from build123d import *

# Parameters (mm, degrees)
SALIENTE_EXTRUIR1_DEPTH                              = 15
CROQUIS2_R                                           = 1.5
CORTAR_EXTRUIR1_DEPTH                                = 5
AVELLANADO_PARA_TORNILLO_CON_CABEZA_PLAN_D           = 3.4
AVELLANADO_PARA_TORNILLO_CON_CABEZA_PLAN_CSINK_D     = 6.3
AVELLANADO_PARA_TORNILLO_CON_CABEZA_PLAN_CSINK_ANGLE = 90


with BuildPart() as part:
    # Croquis1 → Saliente-Extruir1 (new body)
    with BuildSketch(Plane.XY):
        Polygon((-24.277819577, -18.779195804), (-24.277819577, -23.779195804), (-44.277819577, -23.779195804), (-44.277819577, 10.220804196), (-84.277819577, 10.220804196), (-84.277819577, 12.320804196), (-42.177819577, 12.320804196), (-42.177819577, -18.779195804), align=None)
    extrude(amount=SALIENTE_EXTRUIR1_DEPTH)

    # Croquis2 → Cortar-Extruir1 (cut)
    with BuildSketch(Plane(origin=(0, -18.779195804, 0), x_dir=(1, 0, 0), z_dir=(0, 1, 0))):
        with Locations((-33.227819577, -7.5)):
            Circle(CROQUIS2_R)
    extrude(amount=-CORTAR_EXTRUIR1_DEPTH, mode=Mode.SUBTRACT)

    # Avellanado para tornillo con cabeza plana avellanada de M31 (through all)
    with Locations(Plane(origin=(0, -18.779195804, 0), x_dir=(1, 0, 0), z_dir=(0, 1, 0))):
        with Locations((-33.227819577, -7.5)):
            CounterSinkHole(AVELLANADO_PARA_TORNILLO_CON_CABEZA_PLAN_D / 2, AVELLANADO_PARA_TORNILLO_CON_CABEZA_PLAN_CSINK_D / 2, counter_sink_angle=AVELLANADO_PARA_TORNILLO_CON_CABEZA_PLAN_CSINK_ANGLE)


solid = part.part
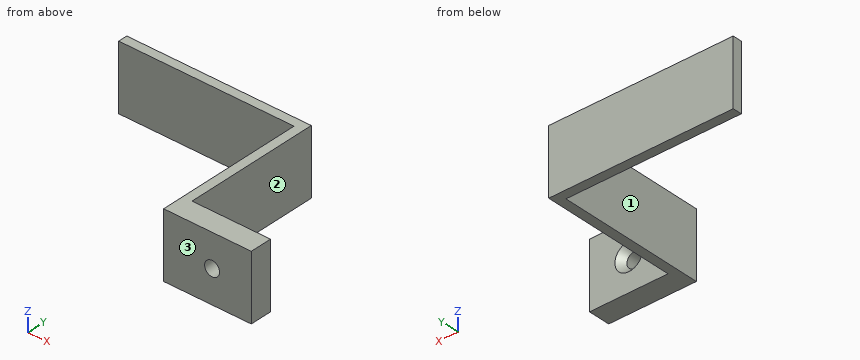
CAD build for the part. Positions are in the model's coordinates, mm. Face numbers are marked on the shaded views. A direction names the side the tool comes from. Give positions to 0.01 mm unless a question says otherwise; leave off trailing zeros. Order: outer loops, then holes, each group sorted by start corner. A loop starts at its lowest first (then second) coordinate and runs counter-clockwise, first axis right, second up. Notation, with made-up numbers: (2, -29) -> (58, -29) arc R29 cw to (58, 1) -> close; hole circle Ø2 at (2.25, -2.75). An arc over 180 degrees is marked (long way). Return JSON: item names as keys, results as strings.
Q1. Flat gauge pins, fed straight in: pin 1 (7.5 mm diameter, centred on y = -5, z = 6.5, fed in from -X); pin 2 (7.5 mm diameter, centred on y = 3, z = 8, fed in from +X); pin 3 (12 mm diameter, centred on x = -61.5, y = 5.5, fed in from +Z); pin 4 (7.5 mm diameter, centred on x = -32, z = 10.5, fed in from +Y). Where does each tip first touch, or does it go through?
Working result:
{"pin 1": "x = -44.28", "pin 2": "x = -42.18", "pin 3": "z = 15", "pin 4": "y = -18.78"}
Q2. Saw through at D-D (x = -70.5). Write the cut outline in (y, z).
Working result:
{"outline": "(10.22, 0) -> (12.32, 0) -> (12.32, 15) -> (10.22, 15) -> close"}
Q3. Drill centre lines: line 1 (X direction, y = -21.15, z = 7.5); line 2 (X direction, y = 0, z = 11.25); line 3 (Y direction, x = -79, z = 4.5). Where is each one in solid material? Low to high.
Working result:
{"line 1": "-44.28 to -34.93, -31.53 to -24.28", "line 2": "-44.28 to -42.18", "line 3": "10.22 to 12.32"}
Q4. Which spindle directions (+Z, -Z, +X, -X, +Y, -Y) get a long thin tool onto all of the face, cutting with end or side? Do the marked faces 1, 2 and 3. Say none if no direction does.
Working result:
{"face 1": "+Z, -Z, -X, -Y", "face 2": "+Z, -Z, +X, +Y", "face 3": "+Z, -Z, +X, -X, -Y"}
Q5. Saw through at A-A (z = 7.5). Write the cut outline in (x, y).
Working result:
{"outline": "(-84.28, 10.22) -> (-44.28, 10.22) -> (-44.28, -23.78) -> (-34.93, -23.78) -> (-34.93, -20.23) -> (-36.38, -18.78) -> (-42.18, -18.78) -> (-42.18, 12.32) -> (-84.28, 12.32) -> close; (-31.53, -23.78) -> (-24.28, -23.78) -> (-24.28, -18.78) -> (-30.08, -18.78) -> (-31.53, -20.23) -> close"}
Q6. Saw through at C-C (z = 11.5). Write the cut outline in (x, y).
Working result:
{"outline": "(-84.28, 10.22) -> (-44.28, 10.22) -> (-44.28, -23.78) -> (-24.28, -23.78) -> (-24.28, -18.78) -> (-42.18, -18.78) -> (-42.18, 12.32) -> (-84.28, 12.32) -> close"}
Q7. Saw through at B-B (y = -21). Write the cut outline in (x, z).
Working result:
{"outline": "(-44.28, 0) -> (-24.28, 0) -> (-24.28, 15) -> (-44.28, 15) -> close; hole circle Ø3.4 at (-33.23, 7.5)"}
